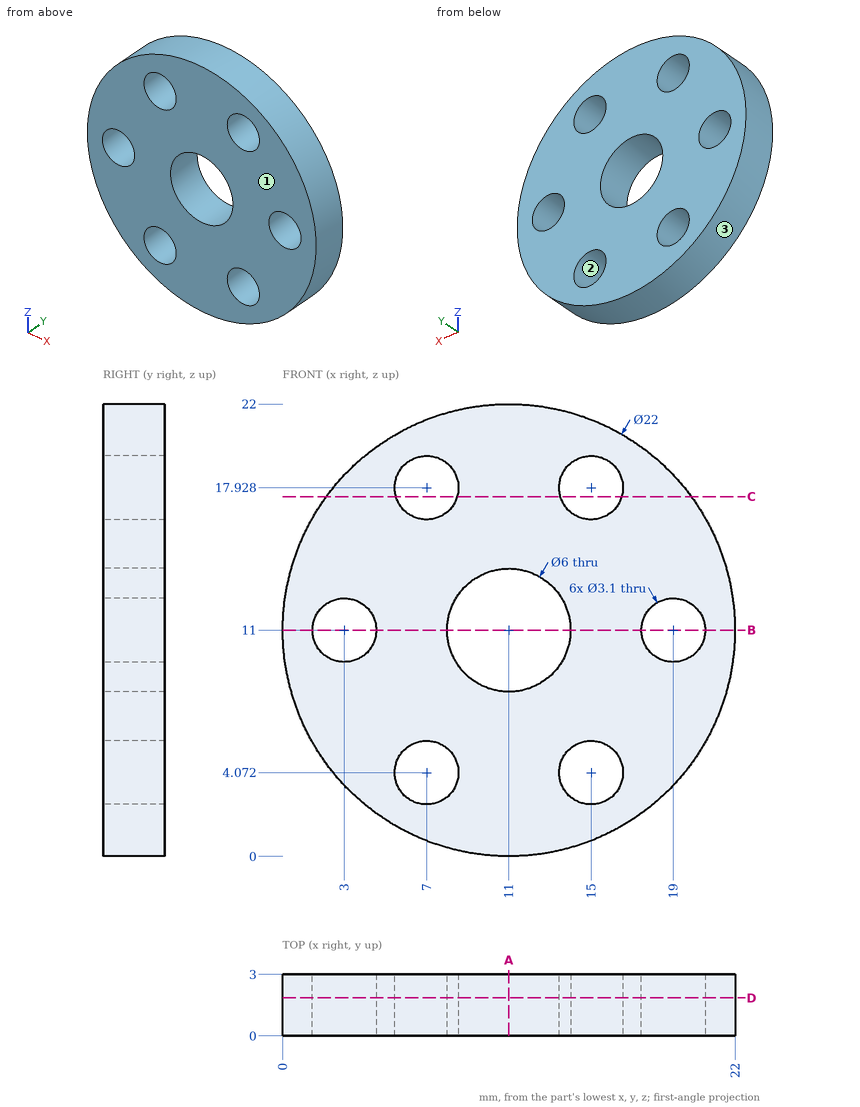
Here's the drawing with two shaded views (mm, measured from the low corner). I have some questions. Coordinates: 2 decimals unless noted, no trailing zeros. Write each loop counter-clockwise with the first axis right and the second up, starting at its lowest first coordinate (ties: lowest second). Pieces come first, ordered by that corner, then holes. Notation, with made-up numbers: (-6.75, 45) -> (2.25, 45) arc R23 cw to (2.25, 64) -> close; hole circle Ø5 at (28.5, 52.5). An arc over 180 degrees is marked (long way). Use a Markdown table: item, result. Add a question column.
(1) If we section it at B-B, the plane z = 11: Write out the boundary of the cut face in (x, y).
(2) If we section it at D-D, the plane y = 1.85: Write out the boundary of the cut face in (x, z), and give its area (3 significant figures).
(3) Please list where these lines run through material, in increasing order: line 1 (Z direction, x = 11, y = 2.2); line 2 (Z direction, x = 16.25, y = 1.15) (1 decimal); line 3 (Z direction, x = 16, y = 2.3) (1 decimal).
(4) If we section it at C-C, the plane z = 17.5: Write out the boundary of the cut face in (x, y).
(5) If we section it at A-A, the plane x = 11: Write out the boundary of the cut face in (y, z).
(6) We'd pull the mould along Z, two halves only. Please class the marked faces 1, 2 and 3: +Z half, -Z half, draft (parallel to the pull), parting line (faces both ways), or undercut.
Outcome:
| question | item | result |
|---|---|---|
| 1 | outline | (0, 0) -> (1.45, 0) -> (1.45, 3) -> (0, 3) -> close; (4.55, 0) -> (8, 0) -> (8, 3) -> (4.55, 3) -> close; (14, 0) -> (17.45, 0) -> (17.45, 3) -> (14, 3) -> close; (20.55, 0) -> (22, 0) -> (22, 3) -> (20.55, 3) -> close |
| 2 | outline | circle Ø22 at (11, 11); hole circle Ø3.1 at (3, 11); hole circle Ø3.1 at (7, 4.07); hole circle Ø3.1 at (7, 17.93); hole circle Ø6 at (11, 11); hole circle Ø3.1 at (15, 4.07); hole circle Ø3.1 at (15, 17.93); hole circle Ø3.1 at (19, 11) |
| 2 | area | 307 mm^2 |
| 3 | line 1 | z = 0 to 8, 14 to 22 |
| 3 | line 2 | z = 1.3 to 3.2, 5 to 17, 18.8 to 20.7 |
| 3 | line 3 | z = 1.2 to 2.9, 5.3 to 16.7, 19.1 to 20.8 |
| 4 | outline | (2.13, 0) -> (5.51, 0) -> (5.51, 3) -> (2.13, 3) -> close; (8.49, 0) -> (13.51, 0) -> (13.51, 3) -> (8.49, 3) -> close; (16.49, 0) -> (19.87, 0) -> (19.87, 3) -> (16.49, 3) -> close |
| 5 | outline | (0, 0) -> (3, 0) -> (3, 8) -> (0, 8) -> close; (0, 14) -> (3, 14) -> (3, 22) -> (0, 22) -> close |
| 6 | face 1 | draft |
| 6 | face 2 | undercut |
| 6 | face 3 | parting line |
